from build123d import *

# Parameters (mm, degrees)
BOSS_EXTRUDE1_DEPTH = 1.8
SKETCH2_W           = 10
SKETCH2_H           = 4
BOSS_EXTRUDE2_DEPTH = 5
SKETCH3_R           = 1.5
CUT_EXTRUDE1_DEPTH  = 5
FILLET1_R           = 2
FILLET2_R           = 0.4


with BuildPart() as part:
    # Sketch1 → Boss-Extrude1 (new body)
    with BuildSketch(Plane(origin=(0, 0, 0), x_dir=(1, 0, 0), z_dir=(0, 1, 0))):
        Polygon((20, 0), (30, 0), (30, -40), (0, -40), (0, 0), (10, 0), (10, 20), (20, 20), align=None)
    extrude(amount=BOSS_EXTRUDE1_DEPTH)

    # Sketch2 → Boss-Extrude2 (add)
    with BuildSketch(Plane(origin=(0, 1.8, 0), x_dir=(1, 0, 0), z_dir=(0, 1, 0))):
        with Locations((15, 18)):
            Rectangle(SKETCH2_W, SKETCH2_H)
    extrude(amount=BOSS_EXTRUDE2_DEPTH)

    # Sketch3 → Cut-Extrude1 (cut)
    with BuildSketch(Plane(origin=(0, 0, -20), x_dir=(-1, 0, 0), z_dir=(0, 0, -1))):
        with Locations((-15, 3.8)):
            Circle(SKETCH3_R)
    extrude(amount=-CUT_EXTRUDE1_DEPTH, mode=Mode.SUBTRACT)

    # Fillet1
    # the kernel refuses this fillet: 2 mm, written as the material it adds along each edge
    with BuildSketch(Plane(origin=(20, 1.8, -16), x_dir=(0, 0, 1), z_dir=(-1, 0, 0))) as fillet1_piece_1_section:
        with BuildLine():
            CenterArc((FILLET1_R, FILLET1_R), FILLET1_R, 180, 90)
            Line((0, FILLET1_R), (0, 0))
            Line((0, 0), (FILLET1_R, 0))
        make_face()
    fillet1_piece_1 = extrude(amount=10, mode=Mode.PRIVATE)
    fillet1_piece_1 = fillet1_piece_1 - Plane(origin=(15, 3.8, -15.523581598), x_dir=(-1, 0, 0), z_dir=(0, 0, -1)) * Cylinder(1.5, 28, mode=Mode.PRIVATE)
    add(fillet1_piece_1)

    # Fillet2
    fillet2_edges = [part.edges().sort_by_distance(p)[0] for p in [
        (15, 0, -20),
    ]]
    fillet(fillet2_edges, radius=FILLET2_R)


solid = part.part
Verification items for the finished model (mm, model axes). A direction names the side the tool comes from. Round coordinates to 2 decimals unless told otherwise and drop trailing zeros. Write each loop counter-clockwise with the first axis right and the second up, starting at its lowest first coordinate (ties: lowest second). Pieces come first, ordered by that corner, then holes.
(1) Access from +Z, -Z, +X, -X, +Y, -Y to the whole of each face (thin tool, end or side, straight path). Record for faces 1 (the flat face through (15, 1.8, 19)), 2 (the flat face through (15, 0, 16)), 3 (the flat face through (30, 1, 20)), 4 (the flat face through (25, 1, 0)), 5 (the flat face through (5, 1, 0)).
Returned:
face 1: +Z, +X, -X, +Y
face 2: +Z, -Z, +X, -X, -Y
face 3: +Z, -Z, +X, +Y, -Y
face 4: -Z, +X, +Y, -Y
face 5: -Z, -X, +Y, -Y
(2) Mould release check, pull along X, two halves, no side actions. Record for faces 6 (the flat face through (15, 2, -20)), 7 (the flat face through (20, 1, -14)), 8 (the cylindrical face through (15.325, 2.336, -17.694)): pulls with the +X half, pulls with the -X half, needs draft (parallel to the pull), parting line crosses it, or undercut.
Returned:
face 6: needs draft
face 7: pulls with the +X half
face 8: undercut
(3) Section check C-C (x = 22.5). Enter the section's corners in (y, z), plus the area to 3 significant figures.
Returned:
outline: (0, 0) - (1.8, 0) - (1.8, 40) - (0, 40) - close
area: 72.0 mm2
(4) Depth check by flat-ended pin: pin 1 Ø1.5 at (x, y) = (16.5, 5.5) entering from +Z; pin 2 Ø3.5 at (y, z) = (4.5, -15) entering from -X; pin 3 Ø15 at (x, z) = (8.5, 4) entering from +Y. Enter the tip coordinate at first touch or a pass-through.
Returned:
pin 1: stops at z = -16
pin 2: stops at x = 10
pin 3: stops at y = 1.8
(5) Section check B-B (z = 27). Enter the section's corners in (x, y), plus the area to 3 significant figures.
Returned:
outline: (0, 0) - (30, 0) - (30, 1.8) - (0, 1.8) - close
area: 54.0 mm2
(6) Section check A-A (x = 15). Enter the section's corners in (y, z), plus the area to 3 significant figures.
Returned:
outline: (0, -19.6) arc R0.4 ccw to (0.4, -20) - (2.3, -20) - (2.3, -15.32) arc R2 cw to (1.8, -14) - (1.8, 40) - (0, 40) - close; (5.3, -20) - (6.8, -20) - (6.8, -16) - (5.3, -16) - close
area: 117 mm2
(7) Material ranges on line 1 (Y direction, x = 15, z = -17.5); line 2 (X direction, y = 3.8, z = -17.85); line 3 (Y direction, x = 5, z = 22.5), recorded low to high.
Returned:
line 1: y = 0 to 2.3, 5.3 to 6.8
line 2: x = 10 to 13.5, 16.5 to 20
line 3: y = 0 to 1.8
